Could you check a few things on this drawing? It's one solid part, dimensions in mm from its lowest x, y, z. A direction names the side the tool comes from. Give positions to 0.01 mm unless a question says otherwise; leave off trailing zeros. Loops run counter-clockwise (first coordinate to the right, second up) from the corner with the lowest first, then second, coordinate; pieces in that order, holes last.
1. For the marked faces 4 and 5, which set-ups out of +Z, -Z, +X, -X, +Y, -Y let a thin tool reach every point of the face, with its end or its side?
2. I need wall thicknesses on line 1 along X through (y, z) = (8.75, 2.55) (3 decimals); line 2 along X through (y, z) = (5, 3.1) (3 decimals); line 3 along Y through (x, z) = (5.5, 1.6). Which ranges of each line are inside material? Lowest first, please.
3. Imagine slicing it at C-C (z = 3.3). List the corners of the cut face in (x, y) for me (3 decimals), plus the area to 3 significant figures.
4. Imagine slicing it at D-D (y = 2.5). List the corners of the cut face in (x, z) for me (3 decimals), plus the area to 3 significant figures.
5. For P1, Ø1, axis at y = 8, z = 2, coming from the +X side; P2, Ø2, axis at x = 9, z = 1, coming from the -Y side; P3, Ø1, axis at y = 7.5, z = 3, coming from the -X side; P4, Ø2, axis at x = 8.5, y = 7.5, coming from the +Z side, each with a flat end and sliding along its axis, tell me the tip position at first contact or that it passes through.
6. Imagine slicing it at A-A (x = 5.75). List the corners of the cut face in (y, z) for me.
7. Thinking about a two-plate mould opening in Y: for the marked faces 1, 2 and 3, which applies, +Y half, -Y half, draft (parallel to the pull), parting line (faces both ways), or undercut?
8. Imagine slicing it at B-B (y = 6). List the corners of the cut face in (x, z) for me (3 decimals), plus the area to 3 significant figures.
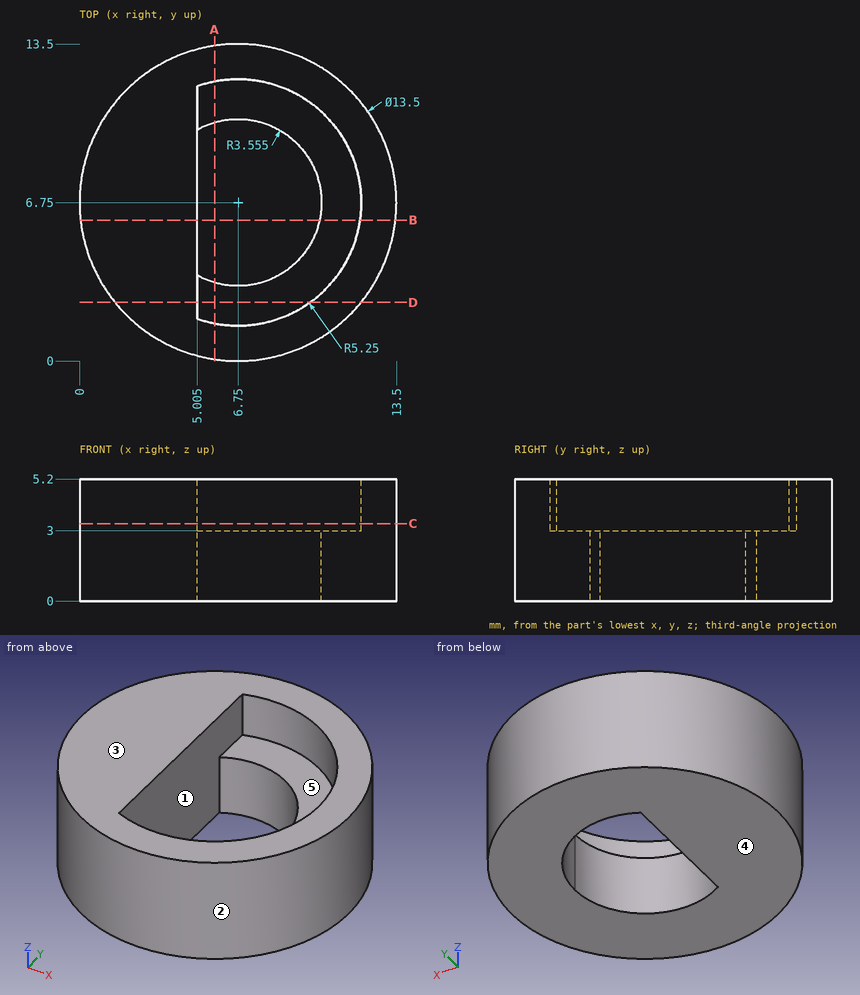
Derived:
1. face 4: -Z, +X, -X, +Y, -Y
1. face 5: +Z
2. line 1: x = 0.303 to 5.005, 9.689 to 13.197
2. line 2: x = 0.231 to 5.005, 11.7 to 13.269
2. line 3: y = 0.12 to 3.42, 10.08 to 13.38
3. outline: circle Ø13.5 at (6.75, 6.75); hole (5.005, 1.798) arc R5.25 ccw (long way) to (5.005, 11.702) - close
3. area: 81.9 mm2
4. outline: (1.506, 0) - (11.994, 0) - (11.994, 5.2) - (9.832, 5.2) - (9.832, 3) - (5.005, 3) - (5.005, 5.2) - (1.506, 5.2) - close
4. area: 43.9 mm2
5. P1: stops at x = 13.46
5. P2: stops at y = 0.12
5. P3: stops at x = 0
5. P4: passes through
6. outline: (0.07, 0) - (3.34, 0) - (3.34, 3) - (1.6, 3) - (1.6, 5.2) - (0.07, 5.2) - close; (10.16, 0) - (13.43, 0) - (13.43, 5.2) - (11.9, 5.2) - (11.9, 3) - (10.16, 3) - close
7. face 1: undercut
7. face 2: parting line
7. face 3: draft
8. outline: (0.042, 0) - (5.005, 0) - (5.005, 5.2) - (0.042, 5.2) - close; (10.225, 0) - (13.458, 0) - (13.458, 5.2) - (11.946, 5.2) - (11.946, 3) - (10.225, 3) - close
8. area: 38.8 mm2
